Design review of the part built by this model. Coordinates are the model's own, in mm. Face numbers are marked on the shaded views. A direction names the side the tool comes from. Give positions to 0.01 mm unless a question says otherwise; leave off trailing zeros. Order: outer loops, then holes, each group sorted by start corner. A loop starts at its lowest first (then second) coordinate and runs counter-clockwise, first axis right, second up. Notation, with made-up numbers: M 5.25,46.5 L 49.25,46.5 A8 cw 49.25,54.5 Z; hole C 64.25,-7.5 d6. An arc over 180 degrees is marked long. Answer as a JSON object with one key per item and string values.
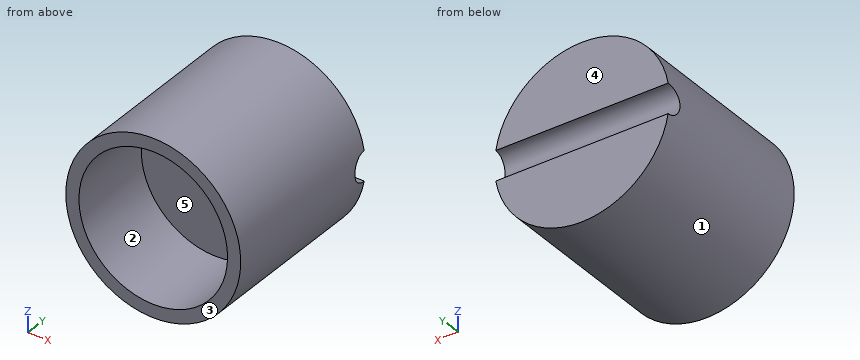
Autodesk Inventor part; units mm, degrees
ref_plane "YZ Plane" through (0, 0, 0) normal (1, 0, 0) x (0, 1, 0)
ref_plane "XZ Plane" through (0, 0, 0) normal (0, 1, 0) x (-1, 0, 0)
ref_plane "XY Plane" through (0, 0, 0) normal (0, 0, 1) x (1, 0, 0)
sketch "Sketch1" plane through (0, 0, 0) normal (0, 1, 0) x (-1, 0, 0)
  circle A0 centre (0, 0) radius 5
  circle A1 centre (0, 0) radius 4.25
  dimension "d0" = 10
  dimension "d1" = 8.5
extrude "Extrusion1" add sketch "Sketch1" along normal blind 10 contours A0 | A1
extrude "Extrusion2" cut sketch "Sketch1" along normal blind 5 contours A1
sketch "Sketch3" plane through (0, 0, 0) normal (1, 0, 0) x (0, 1, 0)
  circle A0 centre (10, 0) radius 0.85
  line L0 (0, -5) -> (10, -5)
  line L1 (0, 5) -> (10, 5)
  line L2 (10, -5) -> (10, 5)
  point P0 (0, 0)
  point P1 (10, -0.85)
  point P2 (10, 0.85)
  dimension "d9" = 1.7
  dimension "d10" = 5
extrude "Extrusion4" cut sketch "Sketch3" along normal mid plane 10 contours L2 A0 picked at (9.5995, 0.1005)
properties part number "rodamiento"
(1) To check wall thickness, follow L1, parallel to Z at x = 0, y = 2.15; L2, parallel to Z at x = 2, y = 2; L3, parallel to X at y = 2.25, z = -2.25. State the ranges of each line that lie inside material, in increasing order. Write a range as from..to.
Checked values:
{"L1": "z = -5..-4.25, 4.25..5", "L2": "z = -4.58..-3.75, 3.75..4.58", "L3": "x = -4.47..-3.61, 3.61..4.47"}
(2) Tool access review of the marked faces 4 and 5: name each direction out of +Z, -Z, +X, -X, +Y, -Y from which nothing blocks a thin tool from reaching the whole face with its end or side.
Checked values:
{"face 4": "+Z, -Z, +X, -X, +Y", "face 5": "-Y"}
(3) We need section C-C (y = 1.5). Write out the cut boundary in (x, z), plus the area to 3 significant figures.
Checked values:
{"outline": "C 0,0 d10; hole C 0,0 d8.5", "area": "21.8 mm^2"}
(4) We need section D-D (y = 9). Write out the cut boundary in (x, z), plus the area to 3 significant figures.
Checked values:
{"outline": "C 0,0 d10", "area": "78.5 mm^2"}
(5) Insertion check: pin 1 (2.5 mm diameter, centred on x = 0.5, z = 1.5, fed in from -Y); pin 2 (2 mm diameter, centred on x = -2.5, y = 8, fed in from +Z); pin 3 (1.5 mm diameter, centred on x = -2.5, y = 1, fed in from +Z). Each pin has a flat end and moves straight along its axis. Give the tip position at first contact, or say it passes through.
Checked values:
{"pin 1": "stops at y = 5", "pin 2": "stops at z = 4.77", "pin 3": "stops at z = 4.68"}
(6) Draft analysis for pull direction Z (two halves, no side actions). For the marked faces 1, 2 and 3, state which applies: +Z half, -Z half, draft (parallel to the pull), parting line (faces both ways), or undercut.
Checked values:
{"face 1": "parting line", "face 2": "undercut", "face 3": "draft"}
(7) We need section A-A (z = 0). Write out the cut boundary in (x, y), plus the area to 3 significant figures.
Checked values:
{"outline": "M -5,0 L -4.25,0 L -4.25,5 L 4.25,5 L 4.25,0 L 5,0 L 5,9.15 L -5,9.15 Z", "area": "49.0 mm^2"}
(8) We need section B-B (x = 0). Write out the cut boundary in (y, z), plus the area to 3 significant figures.
Checked values:
{"outline": "M 0,-5 L 10,-5 L 10,-0.85 A0.85 cw 10,0.85 L 10,5 L 0,5 L 0,4.25 L 5,4.25 L 5,-4.25 L 0,-4.25 Z", "area": "56.4 mm^2"}
